For this review, take the finished solid that the model builds, in its own axes (mm). A direction names the side the tool comes from. Give positions to 0.01 mm unless a question says otherwise; leave off trailing zeros. Write each loop counter-clockwise with the first axis right and the second up, starting at its lowest first coordinate (ties: lowest second). Pieces come first, ordered by that corner, then holes.
Q1. Mouldability with a two-part tool opening along X and no side actions: class faces 1 (the cylindrical face through (24.223, -25.851, 0.231)), 2 (the flat face through (-10, -22.5, 38)), 3 (the cylindrical face through (12.172, 23.243, 12.5)), 4 (the cylindrical face through (18.047, 18.109, 0.231)) as released by +X, released by -X, zero draft, split by the parting line, or undercut.
Q2. Machinability: for faces 5 (the flat face through (1, -5, 59.51)), 6 (the flat face through (19.25, 0, 0)), 7 (the conical face through (9.89, -27.48, 9.86)), 8 (the cylindrical face through (-12.053, -23.243, 11.82)), 9 (the flat face through (8, -22.45, 22)), which of the approach directions +Z, -Z, +X, -X, +Y, -Y give a long, thin tool a straight path to every point of the face, cutting with its end or side? Answer none if there is none.
Q3. Insertion check: P1, Ø4, axis at y = -28, z = 40, coming from the +X side; P2, Ø4, axis at x = 0, y = 0, coming from the -Z side; P3, Ø12.5, axis at x = 7.5, y = 11, coming from the -Z side; P4, Ø1, axis at y = 4, z = 53.5, coming from the +X side. Each pin has a flat end and moves straight along its axis. Give the tip position at first contact, or say it passes through.
Q4. We need section C-C (z = -8). Write out the cut boundary in (x, y), then the cut area to 3 significant figures.
Q5. We need section A-A (y = -23.5). Write out the cut boundary in (x, z) (3 decimals), then the cut area to 3 significant figures.
Q6. For line 1 (Y direction, x = 23, z = -2); line 2 (Y direction, x = 10, z = -10.5); line 3 (Y direction, x = -5, z = 39), list the stretches that pass through material, from the lowest coordinate up.
Q7. We need section D-D (y = 0). Write out the cut boundary in (x, z).
Q8. We need section B-B (y = 13.5). Write out the cut boundary in (x, z).
```python
from build123d import *

# Parameters (mm, degrees)
BOSS_EXTRUDE1_DEPTH                             = 16.51
M5_CLEARANCE_HOLE1_D                            = 5.3
FILLET1_R                                       = 4
BOSS_EXTRUDE2_DEPTH                             = 43
CUT_EXTRUDE1_DEPTH                              = 83.423844244
CUT_EXTRUDE1_DEPTH_BACK                         = 83.423844244
SKETCH7_W                                       = 10
SKETCH7_H                                       = 44.899888642
FILLET2_R                                       = 4
BOSS_EXTRUDE3_START                             = 3
SKETCH8_R                                       = 3.5
BOSS_EXTRUDE3_DEPTH                             = 3
CSK_FOR_M5_FLAT_HEAD_MACHINE_SCREW1_D           = 5.3
CSK_FOR_M5_FLAT_HEAD_MACHINE_SCREW1_DEPTH       = 10.75
CSK_FOR_M5_FLAT_HEAD_MACHINE_SCREW1_CSINK_D     = 10.6
CSK_FOR_M5_FLAT_HEAD_MACHINE_SCREW1_CSINK_ANGLE = 90


with BuildPart() as part:
    # Sketch1 → Boss-Extrude1 (new, symmetric)
    with BuildSketch(Plane.XY):
        Polygon((-19.25, 19.25), (-19.25, 30), (29.25, 30), (29.25, -30), (-19.25, -30), (-19.25, -19.25), (19.25, -19.25), (19.25, 19.25), align=None)
    extrude(amount=BOSS_EXTRUDE1_DEPTH, both=True)

    # M5 Clearance Hole1 (through all)
    with Locations(Plane(origin=(0, 0, -16.51), x_dir=(-1, 0, 0), z_dir=(0, 0, -1))):
        with Locations((-23, -23.5), (-23, 23.5)):
            Hole(M5_CLEARANCE_HOLE1_D / 2)

    # Fillet1
    fillet1_edges = [part.edges().sort_by_distance(p)[0] for p in [
        (19.25, 19.25, 0),
        (29.25, 30, 0),
        (29.25, -30, 0),
        (19.25, -19.25, 0),
    ]]
    fillet(fillet1_edges, radius=FILLET1_R)

    # Sketch6 → Boss-Extrude2 (add)
    with BuildSketch(Plane.XY.offset(16.51)):
        with BuildLine():
            Line((-19.25, 22.5), (-19.25, 30))
            Line((-19.25, 30), (15, 30))
            Line((15, 30), (15, 22.449944321))
            ThreePointArc((15, 22.449944321), (27, 0), (15, -22.449944321))
            Line((15, -22.449944321), (15, -30))
            Line((15, -30), (-19.25, -30))
            Line((-19.25, -30), (-19.25, -22.5))
            Line((-19.25, -22.5), (0, -22.5))
            ThreePointArc((0, -22.5), (22.5, 0), (0, 22.5))
            Line((0, 22.5), (-19.25, 22.5))
        make_face()
    extrude(amount=BOSS_EXTRUDE2_DEPTH)

    # Sketch7 → Cut-Extrude1 (cut, two sides: drawn at the far end of the back side and taken through both)
    with BuildSketch(Plane(origin=(29.25, 0, 0), x_dir=(0, 0, -1), z_dir=(1, 0, 0)).offset(-CUT_EXTRUDE1_DEPTH_BACK)):
        with Locations((-21.51, 0)):
            Rectangle(SKETCH7_W, SKETCH7_H)
    extrude(amount=CUT_EXTRUDE1_DEPTH + CUT_EXTRUDE1_DEPTH_BACK, mode=Mode.SUBTRACT)

    # Fillet2
    fillet2_edges = [part.edges().sort_by_distance(p)[0] for p in [
        (15, -22.449944321, 43.01),
        (15, 22.449944321, 43.01),
    ]]
    fillet(fillet2_edges, radius=FILLET2_R)

    # Sketch8 → Boss-Extrude3 (add)
    with BuildSketch(Plane.XY.offset(59.51).offset(BOSS_EXTRUDE3_START)):
        with BuildLine():
            Line((-19.25, 22.5), (-19.25, -22.5))
            Line((-19.25, -22.5), (-19.25, -30))
            Line((-19.25, -30), (15, -30))
            Line((15, -30), (15, -24.494897428))
            ThreePointArc((15, -24.494897428), (15.407893959, -22.735132048), (16.548387097, -21.334265502))
            ThreePointArc((16.548387097, -21.334265502), (27, 0), (16.548387097, 21.334265502))
            ThreePointArc((16.548387097, 21.334265502), (15.407893959, 22.735132048), (15, 24.494897428))
            Line((15, 24.494897428), (15, 30))
            Line((15, 30), (-19.25, 30))
            Line((-19.25, 30), (-19.25, 22.5))
        make_face()
        Circle(SKETCH8_R, mode=Mode.SUBTRACT)
    extrude(amount=-BOSS_EXTRUDE3_DEPTH)

    # CSK for M5 Flat Head Machine Screw1
    with Locations(Plane(origin=(0, 30, 0), x_dir=(1, 0, 0), z_dir=(0, 1, 0))):
        with Locations((-9.525, -12.61625), (9.525, -12.61625)):
            csk_for_m5_flat_head_machine_screw1 = CounterSinkHole(CSK_FOR_M5_FLAT_HEAD_MACHINE_SCREW1_D / 2, CSK_FOR_M5_FLAT_HEAD_MACHINE_SCREW1_CSINK_D / 2, depth=CSK_FOR_M5_FLAT_HEAD_MACHINE_SCREW1_DEPTH, counter_sink_angle=CSK_FOR_M5_FLAT_HEAD_MACHINE_SCREW1_CSINK_ANGLE)

    # Mirror1: CSK for M5 Flat Head Machine Screw1 across plane
    add(csk_for_m5_flat_head_machine_screw1.mirror(Plane.ZX), mode=Mode.SUBTRACT)


solid = part.part
```
Computed:
1. face 1: undercut
1. face 2: zero draft
1. face 3: undercut
1. face 4: released by -X
2. face 5: -X
2. face 6: -Z, -X
2. face 7: -Y
2. face 8: +Y, -Y
2. face 9: +X, -X
3. P1: stops at x = 15
3. P2: passes through
3. P3: stops at z = 59.51
3. P4: stops at x = 26.77
4. outline: (-19.25, -30) - (25.25, -30) arc R4 ccw to (29.25, -26) - (29.25, 26) arc R4 ccw to (25.25, 30) - (-19.25, 30) - (-19.25, 19.25) - (15.25, 19.25) arc R4 cw to (19.25, 15.25) - (19.25, -15.25) arc R4 cw to (15.25, -19.25) - (-19.25, -19.25) - close; hole circle Ø5.3 at (23, -23.5); hole circle Ø5.3 at (23, 23.5)
4. area: 1,380 mm2
5. outline: (-19.25, -16.51) - (20.35, -16.51) - (20.35, 16.51) - (15, 16.51) - (15, 26.51) - (15.126, 26.51) - (15.126, 62.51) - (-19.25, 62.51) - close; (25.65, -16.51) - (29.25, -16.51) - (29.25, 16.51) - (25.65, 16.51) - close; hole circle Ø5.3 at (-9.525, 12.616); hole circle Ø5.3 at (9.525, 12.616)
5. area: 2,960 mm2
6. line 1: y = -30 to -26.15, -20.85 to 20.85, 26.15 to 30
6. line 2: y = -30 to -19.25, 19.25 to 30
6. line 3: y = -30 to -22.5, 22.5 to 30
7. outline: (-19.25, 59.51) - (-3.5, 59.51) - (-3.5, 62.51) - (-19.25, 62.51) - close; (3.5, 59.51) - (22.5, 59.51) - (22.5, 26.51) - (27, 26.51) - (27, 62.51) - (3.5, 62.51) - close; (19.25, -16.51) - (29.25, -16.51) - (29.25, 16.51) - (19.25, 16.51) - close
8. outline: (-19.25, 59.51) - (18, 59.51) - (18, 26.51) - (23.38, 26.51) - (23.38, 62.51) - (-19.25, 62.51) - close; (19.25, -16.51) - (29.25, -16.51) - (29.25, 16.51) - (19.25, 16.51) - close
